The listing builds one solid part. Answer for the finished solid, in the listing's coordinates (mm). Face numbers are marked on the shaded views. Coordinates: 2 decimals unless noted, no trailing zeros. Write each loop counter-clockwise with the first axis right and the second up, starting at its lowest first coordinate (ties: lowest second). Pieces come first, ordered by that corner, then holes.
Autodesk Inventor part; units mm, degrees
ref_plane "YZ Plane" through (0, 0, 0) normal (1, 0, 0) x (0, 1, 0)
ref_plane "XZ Plane" through (0, 0, 0) normal (0, 1, 0) x (-1, 0, 0)
ref_plane "XY Plane" through (0, 0, 0) normal (0, 0, 1) x (1, 0, 0)
sketch "Sketch1" plane through (0, 0, 0) normal (0, 1, 0) x (-1, 0, 0)
  circle A0 centre (0, 0) radius 2
  circle A1 centre (0, 0) radius 1
  dimension "d0" = 4
  dimension "d3" = 1
extrude "Extrusion1" add sketch "Sketch1" along normal mid plane 48.3
sketch "Sketch2" plane through (0, 0, 0) normal (0, 0, 1) x (1, 0, 0)
  circle A0 centre (6.1, 8.35) radius 5.5 construction
  line L0 (2, 24.15) -> (-2, 24.15)
  circle A1 centre (-9, 8.35) radius 8.5
  line L1 (-0.875, -5) -> (0.875, -5)
  line L2 (0.875, -5) -> (0.875, 5)
  line L3 (0.875, 5) -> (-0.875, 5)
  line L4 (-0.875, 5) -> (-0.875, -5)
  line L5 (-0.875, -5) -> (0.875, 5)
  line L6 (0.875, -5) -> (-0.875, 5)
  circle A2 centre (6.6, 8.35) radius 6
  line L7 (1, 24.15) -> (1, -24.15)
  line L8 (-2, -24.15) -> (2, -24.15)
  point P0 (0, 0)
  point P1 (0.875, 4.8043)
  point P2 (0.875, 4.7957)
  dimension "d6" = 11
  dimension "d8" = 17
  dimension "d12" = 1.75
  dimension "d13" = 10
  dimension "d18" = 12
  dimension "d20" = 1.5
  dimension "d21" = 1.1
  dimension "d25" = 9
  dimension "d26" = 15.8
extrude "Extrusion2" cut sketch "Sketch2" along normal mid plane 10 contours A1 | A2 L7 | L7 A2
properties part number "Fillament Guide" material "Polypropylene"
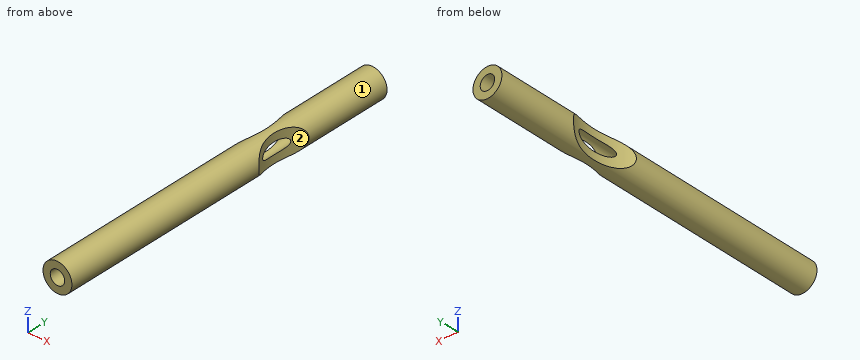
1. Section B-B on z = 0 is taken. Give the vertices of the cut face in (x, y), then the cut area to 3 significant figures.
Results found:
outline: (-2, -24.15) - (-1, -24.15) - (-1, 5.48) arc R8.5 cw to (-2, 3.53) - close; (-2, 13.17) arc R8.5 cw to (-1, 11.22) - (-1, 24.15) - (-2, 24.15) - close; (1, -24.15) - (2, -24.15) - (2, 4.5) arc R6 cw to (1, 6.2) - close; (1, 10.5) arc R6 cw to (2, 12.2) - (2, 24.15) - (1, 24.15) - close
area: 82.5 mm2
2. Find the intervals of material crossed by L1, parallel to Z at x = -0.05, y = 4; L2, parallel to Z at x = 0.4, y = 9.5, in increasing order.
Results found:
L1: z = -2 to -1, 1 to 2
L2: z = -1.96 to -0.92, 0.92 to 1.96
3. Section C-C on y = 18 is taken. Give the vertices of the cut face in (x, z), then the cut area to 3 significant figures.
Results found:
outline: circle Ø4 at (0, 0); hole circle Ø2 at (0, 0)
area: 9.42 mm2
4. For a pull along Y with two mould halves and no side action, classify the marked faces 1 and 2 as pulls with the +Y half, pulls with the -Y half, needs draft (parallel to the pull), parting line crosses it, or undercut.
Results found:
face 1: needs draft
face 2: undercut
5. Section A-A on x = 0 is taken. Give the vertices of the cut face in (y, z), then the cut area to 3 significant figures.
Results found:
outline: (-24.15, -2) - (24.15, -2) - (24.15, -1) - (-24.15, -1) - close; (-24.15, 1) - (24.15, 1) - (24.15, 2) - (-24.15, 2) - close
area: 96.6 mm2
